Geometry: final body of the model. Coordinates: model frame, mm. A direction names the side the tool comes from. Round coordinates to 2 decimals unless told otherwise and drop trailing zeros. Loops run counter-clockwise (first coordinate to the right, second up) from the corner with the lowest first, then second, coordinate; pieces in that order, holes last. Notation, with made-up numbers: (-2, 8.25) - (28, 8.25) arc R20 cw to (28, 46.25) - close; hole circle Ø8 at (55, 38.25). An arc over 180 degrees is marked (long way). Write item = value, one per line. Start each with the question number.
Item 1: Section D-D (z = 19). Return loops of the section in (x, y).
Item 2: Draft query along X for faces 3 (the flat face through (-29, 11, 7)), 4 (the flat face through (0, -11, 0)), 5 (the cylindrical face through (-21.75, 5.69, 6.9)). Return one class per face: pulls with the +X half, pulls with the -X half, needs draft (parallel to the pull), parting line crosses it, or undercut.
Item 3: Section B-B (x = -17.5). Return loops of the section in (y, z).
Item 4: Access query for faces 1 (the flat face through (0, 10.5, 7)), 2 (the flat face through (31.5, 0, 7)). Directions: +Z, -Z, +X, -X, +Y, -Y. A direction counts if a zero-diameter tool reaches every point of the face in a straight line with its end or side. Return the directions, or none.
Item 5: First-contact query: pin 1 (7 mm diameter, centred on x = -23.9, y = -4.6, fed in from +Z); pin 2 (3.5 mm diameter, centred on x = 0, z = 19, fed in from +Y). Flat tips, straight axial feed; report the tip coordinate or a pass-through.
Item 6: Line query: line 1 (Y direction, x = 23.9, z = 10.75); line 2 (Y direction, x = -5, z = 4.75); line 3 (Z direction, x = 0, y = -11.75). Output: solid intervals per line, ascending. Write a range as from..to.
Item 7: Section C-C (y = -4.6). Return loops of the section in (x, z).
Item 8: Section A-A (x = 0). Return loops of the section in (y, z).
from build123d import *

# Parameters (mm, degrees)
SKETCH1_W           = 40
SKETCH1_H           = 21
BOSS_EXTRUDE1_DEPTH = 14
SKETCH2_R           = 2.15
CUT_EXTRUDE1_DEPTH  = 15
BOSS_EXTRUDE2_DEPTH = 10
SKETCH4_R           = 1.5
CUT_EXTRUDE3_DEPTH  = 26


with BuildPart() as part:
    # Sketch1 → Boss-Extrude1 (new body)
    with BuildSketch(Plane.XY):
        Polygon((-27.5, 12.5), (-31.5, 8.5), (-31.5, -8.5), (-27.5, -12.5), (27.5, -12.5), (31.5, -8.5), (31.5, 8.5), (27.5, 12.5), align=None)
        Rectangle(SKETCH1_W, SKETCH1_H, mode=Mode.SUBTRACT)
    extrude(amount=BOSS_EXTRUDE1_DEPTH)

    # Sketch2 → Cut-Extrude1 (cut, through all)
    with BuildSketch(Plane(origin=(0, 0, 0), x_dir=(-1, 0, 0), z_dir=(0, 0, -1))):
        with Locations((-23.9, 5.6)):
            Circle(SKETCH2_R)
        with Locations((-23.9, -4.6)):
            Circle(SKETCH2_R)
        with Locations((23.9, 5.6)):
            Circle(SKETCH2_R)
        with Locations((23.9, -4.6)):
            Circle(SKETCH2_R)
    extrude(amount=-CUT_EXTRUDE1_DEPTH, mode=Mode.SUBTRACT)

    # Sketch3 → Boss-Extrude2 (add)
    with BuildSketch(Plane.XY.offset(14)):
        Polygon((-27.5, -12.5), (27.5, -12.5), (29.5, -10.5), (20, -10.5), (-20, -10.5), (-29.290326063, -10.709673937), align=None)
    extrude(amount=BOSS_EXTRUDE2_DEPTH)

    # Sketch4 → Cut-Extrude3 (cut, through all)
    with BuildSketch(Plane.XZ.offset(12.5)):
        with Locations((-20, 19)):
            Circle(SKETCH4_R)
        with Locations((20, 19)):
            Circle(SKETCH4_R)
        with Locations((0, 19)):
            Circle(SKETCH4_R)
    extrude(amount=-CUT_EXTRUDE3_DEPTH, mode=Mode.SUBTRACT)


solid = part.part
Taken from the geometry:
q1.outline = (-29.29, -10.71) - (-27.5, -12.5) - (-21.5, -12.5) - (-21.5, -10.53) - close; (-18.5, -12.5) - (-1.5, -12.5) - (-1.5, -10.5) - (-18.5, -10.5) - close; (1.5, -12.5) - (18.5, -12.5) - (18.5, -10.5) - (1.5, -10.5) - close; (21.5, -12.5) - (27.5, -12.5) - (29.5, -10.5) - (21.5, -10.5) - close
q2.face_3 = pulls with the -X half
q2.face_4 = needs draft
q2.face_5 = undercut
q3.outline = (-12.5, 0) - (-10.5, 0) - (-10.5, 24) - (-12.5, 24) - close; (10.5, 0) - (12.5, 0) - (12.5, 14) - (10.5, 14) - close
q4.face_1 = +Z, -Z
q4.face_2 = +Z, -Z, +X, +Y, -Y
q5.pin_1 = 14
q5.pin_2 = -10.5
q6.line_1 = -12.5..-6.75, -2.45..3.45, 7.75..12.5
q6.line_2 = -12.5..-10.5, 10.5..12.5
q6.line_3 = 0..17.5, 20.5..24
q7.outline = (-31.5, 0) - (-26.05, 0) - (-26.05, 14) - (-31.5, 14) - close; (-21.75, 0) - (-20, 0) - (-20, 14) - (-21.75, 14) - close; (20, 0) - (21.75, 0) - (21.75, 14) - (20, 14) - close; (26.05, 0) - (31.5, 0) - (31.5, 14) - (26.05, 14) - close
q8.outline = (-12.5, 0) - (-10.5, 0) - (-10.5, 17.5) - (-12.5, 17.5) - close; (-12.5, 20.5) - (-10.5, 20.5) - (-10.5, 24) - (-12.5, 24) - close; (10.5, 0) - (12.5, 0) - (12.5, 14) - (10.5, 14) - close
